Can you work these out from the model? Positions are in its coordinate system, mm. A direction names the side the tool comes from. Coordinates: 2 decimals unless noted, no trailing zeros. Order: outer loops, then holes, each group sorted by start corner. A loop starts at its lowest first (then second) coordinate and runs counter-clockwise, first axis right, second up. Notation, with made-up numbers: (-15.5, -13.5) -> (-3.5, -13.5) arc R22 cw to (-3.5, 19.5) -> close; hole circle Ø3 at (-4.75, 80). An arc over 180 degrees is marked (long way). Answer in a Markdown table with one row per item. Add a question column.
1. We'd pull the mould along Y, two halves only. Please class faces 1 (the face through (-86, 134, 767.5)), 2 (the face through (-20.66, 157.35, 764.96)), 3 (the face through (-35.444, -159.612, 10.745)): pulls with the +Y half, pulls with the -Y half, needs draft (parallel to the pull), parting line crosses it, or undercut.
2. Imagine slicing it at C-C on x = 101.5. Write out the boundary of the cut face in (y, z), plus the area to 3 significant figures.
3. Will these pins go through, and if not, where does the flat tip stop? pin 1 (8 mm diameter, centred on x = -14, y = -57, fed in from +Z); pin 2 (5 mm diameter, centred on x = 19, y = -80, fed in from -Z); pin 3 (12 mm diameter, centred on y = 110.5, z = 222, fed in from +X).
4. If I drill on line 1 along Z through (x, y) = (-64, 97); line 2 along X through (y, z) = (0, 858.25); line 3 along Y through (x, z) = (-109.5, 4), over which ranges is the centre line in solid material (lowest first)? Write a range as [from, to].
5. On a 3-axis mill with a long thin cutter (end or side, diameter ignored), from which of +Z, -Z, +X, -X, +Y, -Y can I reach the whole of each face in a straight line? I mean faces 4 (the face through (-20.66, 157.35, -10.61)), 5 (the face through (-2, -33, 762.5)), 6 (the face through (-20.66, 157.35, -765.04)). Say none if no direction works.
6. Imagine slicing it at A-A on z = 486.5. Write out the boundary of the cut face in (x, y), plus the area to 3 significant figures.
7. Imagine slicing it at B-B on y = -61.5. Write out the boundary of the cut face in (x, z), plus the area to 3 significant figures.
from build123d import *

# Parameters (mm, degrees)
SKETCH1_R           = 163.5
SKETCH1_R_2         = 158.7
BOSS_EXTRUDE1_DEPTH = 767.5
BOSS_EXTRUDE2_START = -10
SKETCH2_R           = 158.7
BOSS_EXTRUDE2_DEPTH = 5
CHAMFER1_SIZE       = 0.5


with BuildPart() as part:
    # Sketch1 → Boss-Extrude1 (new, symmetric)
    with BuildSketch(Plane.XY):
        Circle(SKETCH1_R)
        Circle(SKETCH1_R_2, mode=Mode.SUBTRACT)
    extrude(amount=BOSS_EXTRUDE1_DEPTH, both=True)

    # Sketch2 → Boss-Extrude2 (add)
    with BuildSketch(Plane.XY.offset(767.5).offset(BOSS_EXTRUDE2_START)):
        Circle(SKETCH2_R)
    boss_extrude2 = extrude(amount=BOSS_EXTRUDE2_DEPTH)

    # Sketch5 → Revolve1 (revolve)
    with BuildSketch(Plane(origin=(0, 0, 0), x_dir=(0, 0, -1), z_dir=(1, 0, 0)), mode=Mode.PRIVATE) as revolve1_sk:
        Polygon((-782.5, 12), (782.5, 12), (782.5, 10.5), (863.5, 10.5), (863.5, 0), (-863.5, 0), (-863.5, 10.5), (-782.5, 10.5), align=None)
    revolve(revolve1_sk.sketch.rotate(Axis((0, 0, -863.5), (0, 0, -1)), 180), axis=Axis((0, 0, -863.5), (0, 0, -1)))

    # Chamfer1
    chamfer1_edges = [part.edges().sort_by_distance(p)[0] for p in [
        (0, 12, -782.5),
        (0, 12, 782.5),
        (0, 10.5, -863.5),
        (0, 10.5, 863.5),
    ]]
    chamfer(chamfer1_edges, length=CHAMFER1_SIZE)

    # Sketch7 → M6 Tapped Hole1 (revolve, cut)
    with BuildSketch(Plane(origin=(0, 0, 863.5), x_dir=(0, -1, 0), z_dir=(1, 0, 0))):
        Polygon((0, 0), (0, 16.502151548), (2.5, 15), (2.5, 0), align=None)
    m6_tapped_hole1 = revolve(axis=Axis((0, 0, 869.85), (0, 0, -1)), mode=Mode.SUBTRACT)

    # Mirror3: Boss-Extrude2, M6 Tapped Hole1 across plane
    add(boss_extrude2.mirror(Plane.XY))
    add(m6_tapped_hole1.mirror(Plane.XY), mode=Mode.SUBTRACT)


solid = part.part
Answers follow:
| question | item | result |
|---|---|---|
| 1 | face 1 | needs draft |
| 1 | face 2 | undercut |
| 1 | face 3 | parting line crosses it |
| 2 | outline | (-128.18, -767.5) -> (-122, -767.5) -> (-122, -762.5) -> (122, -762.5) -> (122, -767.5) -> (128.18, -767.5) -> (128.18, 767.5) -> (122, 767.5) -> (122, 762.5) -> (-122, 762.5) -> (-122, 767.5) -> (-128.18, 767.5) -> close; hole (-122, -757.5) -> (122, -757.5) -> (122, 757.5) -> (-122, 757.5) -> close |
| 2 | area | 21,400 mm² |
| 3 | pin 1 | stops at z = 762.5 |
| 3 | pin 2 | stops at z = -762.5 |
| 3 | pin 3 | stops at x = 125.75 |
| 4 | line 1 | z = [-762.5, -757.5], [757.5, 762.5] |
| 4 | line 2 | x = [-10.5, -2.5], [2.5, 10.5] |
| 4 | line 3 | y = [-121.42, -114.87], [114.87, 121.42] |
| 5 | face 4 | none |
| 5 | face 5 | +Z |
| 5 | face 6 | -Z |
| 6 | outline | circle Ø327 at (0, 0); circle Ø24 at (0, 0); hole circle Ø317.4 at (0, 0) |
| 6 | area | 5,310 mm² |
| 7 | outline | (-151.49, -767.5) -> (-146.3, -767.5) -> (-146.3, -762.5) -> (146.3, -762.5) -> (146.3, -767.5) -> (151.49, -767.5) -> (151.49, 767.5) -> (146.3, 767.5) -> (146.3, 762.5) -> (-146.3, 762.5) -> (-146.3, 767.5) -> (-151.49, 767.5) -> close; hole (-146.3, -757.5) -> (146.3, -757.5) -> (146.3, 757.5) -> (-146.3, 757.5) -> close |
| 7 | area | 18,900 mm² |
